Could you check a few things on this model? Use its own coordinates, in mm. A direction names the side the tool comes from. Give positions to 0.01 mm unless a question says otherwise; leave off trailing zeros. Loops run counter-clockwise (first coordinate to the right, second up) from the corner with the lowest first, then second, coordinate; pieces in that order, holes last. Notation, with made-up numbers: M 19.5,-19.75 L 38.5,-19.75 A31 cw 38.5,16.25 Z; hole C 46,-1.75 d1. An arc over 180 degrees is marked long. Answer in a Markdown table with one row per item. Add a question column.
```python
from build123d import *

# Parameters (mm, degrees)
F0_W     = 153
F0_H     = 69
F1_DEPTH = 1.7
F2_W     = 15
F2_H     = 4.6
F2_W_2   = 8
F2_W_3   = 1.9
F2_H_2   = 8.5
F2_W_4   = 18.5
F2_H_3   = 12.6
F2_R     = 2
F2_R_2   = 1.7
F2_W_5   = 6.6
F2_H_4   = 2.1
F3_DEPTH = 1.701
F4_W     = 89.7158287823
F4_H     = 5
F5_DEPTH = 1.701
F6_DEPTH = 7.25
F8_DEPTH = 7.251
F9_DEPTH = 0.5


with BuildPart() as f1:
    # F0 (on Top) → F1 (new body)
    with BuildSketch(Plane.XY):
        Rectangle(F0_W, F0_H)
    extrude(amount=F1_DEPTH)

    # F2 (on face) → F3 (cut, through all)
    with BuildSketch(Plane.XY.offset(1.7)):
        with Locations((-69, -32.2)):
            Rectangle(F2_W, F2_H)
        Polygon((-61.5, -29.9), (-61.5, -34.5), (-43.1, -34.5), (-43.1, -29.9), (-43.1, -21.9), (-61.5, -21.9), align=None)
        with Locations((-39.1, -32.2)):
            Rectangle(F2_W_2, F2_H)
        Polygon((-35.1, -29.9), (-35.1, -34.5), (-31.6, -34.5), (-31.6, -21.9), (-35.1, -21.9), align=None)
        with Locations((-19.35, -30.25)):
            Rectangle(F2_W_3, F2_H_2)
        with Locations((67.25, -28.2)):
            Rectangle(F2_W_4, F2_H_3)
        with Locations((-69, -24.9)):
            Circle(F2_R)
        with Locations((-69, 19.1)):
            Circle(F2_R)
        with Locations((71.5, 18.8)):
            Circle(F2_R_2)
        with Locations((71.5, -6.2)):
            Circle(F2_R_2)
        with Locations((41.5, 18.8)):
            Circle(F2_R_2)
        with Locations((41.5, -6.2)):
            Circle(F2_R_2)
        with Locations((-38.5, 29.05)):
            Rectangle(F2_W_5, F2_H_4)
        with Locations((-38.5, 8.55)):
            Rectangle(F2_W_5, F2_H_4)
        with Locations((-38.5, -16.45)):
            Rectangle(F2_W_5, F2_H_4)
        with Locations((-38.5, 4.05)):
            Rectangle(F2_W_5, F2_H_4)
        with Locations((61.5, 29.05)):
            Rectangle(F2_W_5, F2_H_4)
        with Locations((61.5, 8.55)):
            Rectangle(F2_W_5, F2_H_4)
        with Locations((61.5, 4.05)):
            Rectangle(F2_W_5, F2_H_4)
        with Locations((61.5, -16.45)):
            Rectangle(F2_W_5, F2_H_4)
        with Locations((-18.5, 18.8)):
            Circle(F2_R_2)
        with Locations((-48.5, 18.8)):
            Circle(F2_R_2)
        with Locations((-18.5, -6.2)):
            Circle(F2_R_2)
        with Locations((-48.5, -6.2)):
            Circle(F2_R_2)
    extrude(amount=-F3_DEPTH, mode=Mode.SUBTRACT)

    # F4 (on Top) → F5 (cut, through all)
    with BuildSketch(Plane.XY):
        with Locations((13.2579143912, -21.45)):
            Rectangle(F4_W, F4_H)
    extrude(amount=F5_DEPTH, mode=Mode.SUBTRACT)

    # F4 (on Top) → F6 (join)
    with BuildSketch(Plane.XY):
        with Locations((13.2579143912, -21.45)):
            Rectangle(F4_W, F4_H)
    extrude(amount=F6_DEPTH)

    # F7 (on Top) → F8 (cut, through all)
    with BuildSketch(Plane.XY):
        Polygon((76.5, -21.9), (76.5, 34.5), (-76.5, 34.5), (-76.5, -29.9), (-61.5, -29.9), (-61.5, -21.9), (-43.1, -21.9), (-43.1, -29.9), (-35.1, -29.9), (-35.1, -21.9), (-31.6, -21.9), (-31.6, -18.95), (58.1158287823, -18.95), (58.1158287823, -21.9), align=None)
    extrude(amount=F8_DEPTH, mode=Mode.SUBTRACT)

    # F9 (cut): a face of the model
    f9_faces = [f1.faces().sort_by_distance(p)[0] for p in [
        (13.7657792774, -29.2071836019, 1.7),
    ]]
    extrude(f9_faces, amount=-F9_DEPTH, mode=Mode.SUBTRACT)


solid = f1.part
```
Item 1: For faces 1 (the face through (13, -29, 1.2)), 2 (the face through (-31.6, -23, 3)), which set-ups out of +Z, -Z, +X, -X, +Y, -Y let a thin tool reach every point of the face, with its end or its side?
Item 2: Suppose I cut it at B-B (x = 46). List the corners of the cut face in (y, z) for me, then the cut area to 3 significant figures.
Item 3: Suppose I cut it at C-C (z = 6). List the corners of the cut face in (x, y) for me, then the cut area to 3 significant figures.
Item 4: For P1, Ø1.3, axis at y = -29, z = 1, coming from the +X side; P2, Ø5.5, axis at x = 33, y = -29, coming from the +Z side, each with a flat end and sliding along its axis, tell me the tip position at first contact or that it passes through.
Item 5: I need wall thicknesses on L1, parallel to Z at x = 33, y = -30; L2, parallel to Y at x = 15, z = 5.5. Which ranges of each line are inside material? Lowest first, please.
Item 6: Suppose I cut it at A-A (y = -27.75). List the corners of the cut face in (x, z) for me, then the cut area to 3 significant figures.
Values found:
| question | item | result |
|---|---|---|
| 1 | face 1 | +Z, +X, -X, -Y |
| 1 | face 2 | +Z, -Z, -X, +Y, -Y |
| 2 | outline | M -34.5,0 L -18.95,0 L -18.95,7.25 L -23.95,7.25 L -23.95,1.2 L -34.5,1.2 Z |
| 2 | area | 48.9 mm² |
| 3 | outline | M -31.6,-23.95 L 58.12,-23.95 L 58.12,-18.95 L -31.6,-18.95 Z |
| 3 | area | 449 mm² |
| 4 | P1 | x = 58 |
| 4 | P2 | z = 1.2 |
| 5 | L1 | 0 to 1.2 |
| 5 | L2 | -23.95 to -18.95 |
| 6 | outline | M -31.6,0 L -20.3,0 L -20.3,1.2 L -31.6,1.2 Z; M -18.4,0 L 58,0 L 58,1.2 L -18.4,1.2 Z |
| 6 | area | 105 mm² |
